from build123d import *

# Parameters (mm, degrees)
ESQUISSE1_W             = 42
ESQUISSE1_H             = 14
BOSS_EXTRU_1_DEPTH      = 32
ESQUISSE2_W             = 12
ESQUISSE2_H             = 27
ENL_V_MAT_EXTRU_1_DEPTH = 41.755367745
ESQUISSE3_R             = 4
ENL_V_MAT_EXTRU_2_DEPTH = 41.755367745
ESQUISSE4_W             = 1
ESQUISSE4_H             = 13.961299029
ENL_V_MAT_EXTRU_3_DEPTH = 41.755367745
ESQUISSE5_R             = 2.5
ENL_V_MAT_EXTRU_4_DEPTH = 35.9141805


with BuildPart() as part:
    # Esquisse1 → Boss.-Extru.1 (new body)
    with BuildSketch(Plane(origin=(0, 0, 0), x_dir=(1, 0, 0), z_dir=(0, 1, 0))):
        Rectangle(ESQUISSE1_W, ESQUISSE1_H)
    extrude(amount=BOSS_EXTRU_1_DEPTH)

    # Esquisse2 → Enlèv. mat.-Extru.1 (cut, through all)
    with BuildSketch(Plane.XY.offset(7)):
        with Locations((-15, 18.5)):
            Rectangle(ESQUISSE2_W, ESQUISSE2_H)
        with Locations((15, 18.5)):
            Rectangle(ESQUISSE2_W, ESQUISSE2_H)
    extrude(amount=-ENL_V_MAT_EXTRU_1_DEPTH, mode=Mode.SUBTRACT)

    # Esquisse3 → Enlèv. mat.-Extru.2 (cut, through all)
    with BuildSketch(Plane.XY.offset(7)):
        with Locations((0, 20)):
            Circle(ESQUISSE3_R)
    extrude(amount=-ENL_V_MAT_EXTRU_2_DEPTH, mode=Mode.SUBTRACT)

    # Esquisse4 → Enlèv. mat.-Extru.3 (cut, through all)
    with BuildSketch(Plane.XY.offset(7)):
        with Locations((0, 25.019350485)):
            Rectangle(ESQUISSE4_W, ESQUISSE4_H)
    extrude(amount=-ENL_V_MAT_EXTRU_3_DEPTH, mode=Mode.SUBTRACT)

    # Esquisse5 → Enlèv. mat.-Extru.4 (cut, through all)
    with BuildSketch(Plane(origin=(0, 5, 0), x_dir=(1, 0, 0), z_dir=(0, 1, 0))):
        with Locations(Location((-15.75, 1, 0), (0, 0, 270))):
            Circle(ESQUISSE5_R)
        with Locations(Location((15.75, 1, 0), (0, 0, 270))):
            Circle(ESQUISSE5_R)
    extrude(amount=-ENL_V_MAT_EXTRU_4_DEPTH, mode=Mode.SUBTRACT)


solid = part.part
CAD build for the part. Positions are in the model's coordinates, mm. A direction names the side the tool comes from. Give positions to 0.01 mm unless a question says otherwise; leave off trailing zeros. Order: outer loops, then holes, each group sorted by start corner. A loop starts at its lowest first (then second) coordinate and runs counter-clockwise, first axis right, second up. Notation, with made-up numbers: (-31, 80) - (25, 80) arc R35 ccw to (25, 117) - close; hole circle Ø4 at (14, 69.25). An arc over 180 degrees is marked (long way). Answer in a Markdown table with one row per item.
1. Tool access for faces 1 (the flat face through (15, 5, 2)), 2 (the flat face through (-15, 5, 2)), 3 (the flat face through (0.5, 28, 0)): list every direction of +Z, -Z, +X, -X, +Y, -Y with a clear straight run to the whole face (end or side of a thin tool).
Data:
| item | result |
|---|---|
| face 1 | +Z, -Z, +X, +Y |
| face 2 | +Z, -Z, -X, +Y |
| face 3 | +Z, -Z, +Y |
2. Saw through at B-B, the plane x = -15.75. Give the cut face in (y, z).
Data:
| item | result |
|---|---|
| outline | (0, -7) - (5, -7) - (5, -3.5) - (0, -3.5) - close; (0, 1.5) - (5, 1.5) - (5, 7) - (0, 7) - close |
3. Pull direction Z, two halves, no side cores. Call faces 4 (the flat face through (0, 0, 0)), 5 (the flat face through (0, 11, -7)), 6 (the cylindrical face through (13.53, 2.54, 0.15)): pulls with the +Z half, pulls with the -Z half, needs draft (parallel to the pull), parting line crosses it, or undercut.
Data:
| item | result |
|---|---|
| face 4 | needs draft |
| face 5 | pulls with the -Z half |
| face 6 | undercut |
4. Flat gauge pins, fed straight in: pin 1 (6.5 mm diameter, centred on y = 26, z = 1, fed in from -X); pin 2 (5 mm diameter, centred on x = 0, y = 20, fed in from -Z); pin 3 (6.5 mm diameter, centred on y = 26, z = -3.5, fed in from +X); pin 4 (3.5 mm diameter, centred on x = -13.5, z = -2, fed in from +Y). Where does each tip first touch, or does it go through?
Data:
| item | result |
|---|---|
| pin 1 | stops at x = -9 |
| pin 2 | passes through |
| pin 3 | stops at x = 9 |
| pin 4 | stops at y = 5 |
5. Saw through at A-A, the plane y = 20. Give the cut face in (x, z).
Data:
| item | result |
|---|---|
| outline | (-9, -7) - (-4, -7) - (-4, 7) - (-9, 7) - close; (4, -7) - (9, -7) - (9, 7) - (4, 7) - close |
6. Probe probe 1 along X at (y, z) = (3.45, -1); probe 2 along X at (y, z) = (20, -3.25); probe 3 along X at (y, z) = (29, 2.5). List the from-to ranges inside material, lowest first. Write a range as [from, to].
Data:
| item | result |
|---|---|
| probe 1 | x = [-21, -18.25], [-13.25, 13.25], [18.25, 21] |
| probe 2 | x = [-9, -4], [4, 9] |
| probe 3 | x = [-9, -0.5], [0.5, 9] |
7. Saw through at D-D, the plane x = 0. Give the cut face in (y, z), plus the area to 3 significant figures.
Data:
| item | result |
|---|---|
| outline | (0, -7) - (16, -7) - (16, 7) - (0, 7) - close |
| area | 224 mm² |
8. Saw through at C-C, the plane z = -1. Give the cut face in (x, y), plus the area to 3 significant figures.
Data:
| item | result |
|---|---|
| outline | (-21, 0) - (-18.25, 0) - (-18.25, 5) - (-21, 5) - close; (-13.25, 0) - (13.25, 0) - (13.25, 5) - (9, 5) - (9, 32) - (0.5, 32) - (0.5, 23.97) arc R4 cw (long way) to (-0.5, 23.97) - (-0.5, 32) - (-9, 32) - (-9, 5) - (-13.25, 5) - close; (18.25, 0) - (21, 0) - (21, 5) - (18.25, 5) - close |
| area | 588 mm² |
